Can you work these out from the model? Positions are in its coordinate system, mm. A direction names the side the tool comes from. Round coordinates to 2 decimals unless told otherwise and drop trailing zeros. Write each loop counter-clockwise with the first axis right and the second up, starting at its lowest first coordinate (ties: lowest second). Pieces come first, ordered by that corner, then holes. Notation, with made-up numbers: (62, -37) -> (69, -37) arc R13 cw to (69, -19) -> close; hole circle Ø10 at (-24, -38). An arc over 180 degrees is marked (long way). Write item = value, one per line. Start each with the question number.
1) I'm going to push flat-ended pins straight in: pin 1 (2 mm diameter, centred on x = 4, y = -15.5, fed in from +Z); pin 2 (15 mm diameter, centred on y = 1.5, z = 22.5, fed in from +X); pin 3 (1 mm diameter, centred on x = -3.5, z = 30.5, fed in from -Y). Where does each tip first touch, or does it pass through?
2) For faces 5 (the face through (4, -25, 2)), 6 (the face through (-21, -1, 20)), 7 (the face through (21, 4, 19)), which set-ups out of +Z, -Z, +X, -X, +Y, -Y let a thin tool reach every point of the face, with its end or its side?
3) Thinking about a two-plate mould opening in Y: for faces 1 (the face through (-1, 22, 20)), 2 (the face through (-23, 0.2, 18.3)), 3 (the face through (0, 25, 19)), 4 (the face through (-25, 0, 15)), which applies, +Y half, -Y half, draft (parallel to the pull), parting line (faces both ways), or undercut?
4) Imagine slicing it at C-C, the plane x = -2. Please give me the cut outline in (y, z).
5) Imagine slicing it at A-A, the plane z = 21.5. Please give me the cut outline in (x, y), then the cut area to 3 significant figures.
6) If I drill on line 1 (X direction, y = -13, z = 30.5); line 2 (X direction, y = -22, z = 34); line 3 (Z direction, x = 20.6, y = 0), over which ranges is the centre line in solid material (lowest first)?
7) Imagine slicing it at B-B, the plane y = 0. Please give me the cut outline in (x, z), then the cut area to 4 significant figures.
from build123d import *

# Parameters (mm, degrees)
SKETCH8_W            = 50
SKETCH8_H            = 50
BOSS_EXTRUDE7_DEPTH  = 3
SKETCH9_W            = 38
SKETCH9_H            = 50
BOSS_EXTRUDE8_DEPTH  = 5
SKETCH10_W           = 38
SKETCH10_H           = 50
BOSS_EXTRUDE9_DEPTH  = 4
SKETCH11_W           = 50
SKETCH11_H           = 38
BOSS_EXTRUDE10_DEPTH = 3
SKETCH13_W           = 38
SKETCH13_H           = 29.975664986
CUT_EXTRUDE1_DEPTH   = 4
SKETCH14_R           = 0.75
CUT_EXTRUDE3_DEPTH   = 68


with BuildPart() as part:
    # Sketch8 → Boss-Extrude7 (new body)
    with BuildSketch(Plane.XY):
        Rectangle(SKETCH8_W, SKETCH8_H)
    extrude(amount=BOSS_EXTRUDE7_DEPTH)

    # Sketch9 → Boss-Extrude8 (add)
    with BuildSketch(Plane(origin=(25, 0, 0), x_dir=(0, 0, -1), z_dir=(1, 0, 0))):
        with Locations((-19, 0)):
            Rectangle(SKETCH9_W, SKETCH9_H)
    extrude(amount=-BOSS_EXTRUDE8_DEPTH)

    # Sketch10 → Boss-Extrude9 (add)
    with BuildSketch(Plane.ZY.offset(25)):
        with Locations((19, 0)):
            Rectangle(SKETCH10_W, SKETCH10_H)
    extrude(amount=-BOSS_EXTRUDE9_DEPTH)

    # Sketch11 → Boss-Extrude10 (add)
    with BuildSketch(Plane(origin=(0, 25, 0), x_dir=(1, 0, 0), z_dir=(0, 1, 0))):
        with Locations((0, -19)):
            Rectangle(SKETCH11_W, SKETCH11_H)
    extrude(amount=-BOSS_EXTRUDE10_DEPTH)

    # Sketch13 → Cut-Extrude1 (cut)
    with BuildSketch(Plane(origin=(25, 0, 0), x_dir=(0, 0, -1), z_dir=(1, 0, 0))):
        with Locations((-19, 0)):
            Rectangle(SKETCH13_W, SKETCH13_H)
    extrude(amount=-CUT_EXTRUDE1_DEPTH, mode=Mode.SUBTRACT)

    # Sketch14 → Cut-Extrude3 (cut)
    with BuildSketch(Plane.ZY.offset(25)):
        with Locations(Location((19.021319819, 0, 0), (0, 0, 270))):
            Circle(SKETCH14_R)
    extrude(amount=-CUT_EXTRUDE3_DEPTH, mode=Mode.SUBTRACT)


solid = part.part
Reported:
q1.pin_1 = 3
q1.pin_2 = 21
q1.pin_3 = 22
q2.face_5 = +Z, -Z, +X, -X, -Y
q2.face_6 = +Z, -Y
q2.face_7 = +Z, -Z, +X
q3.face_1 = -Y half
q3.face_2 = undercut
q3.face_3 = +Y half
q3.face_4 = draft
q4.outline = (-25, 0) -> (25, 0) -> (25, 38) -> (22, 38) -> (22, 3) -> (-25, 3) -> close
q5.outline = (-25, -25) -> (-21, -25) -> (-21, 22) -> (20, 22) -> (20, -25) -> (25, -25) -> (25, -14.99) -> (21, -14.99) -> (21, 14.99) -> (25, 14.99) -> (25, 25) -> (-25, 25) -> close
q5.area = 453 mm²
q6.line_1 = -25 to -21, 20 to 21
q6.line_2 = -25 to -21, 20 to 25
q6.line_3 = 0 to 18.27, 19.77 to 38
q7.outline = (-25, 0) -> (21, 0) -> (21, 18.27) -> (20, 18.27) -> (20, 3) -> (-21, 3) -> (-21, 18.27) -> (-25, 18.27) -> close; (-25, 19.77) -> (-21, 19.77) -> (-21, 38) -> (-25, 38) -> close; (20, 19.77) -> (21, 19.77) -> (21, 38) -> (20, 38) -> close
q7.area = 305.5 mm²
